```python
from build123d import *

# Parameters (mm, degrees)
F1_DEPTH = 1.27


with BuildPart() as f1:
    # F0 (on Front) → F1 (new body, symmetric)
    with BuildSketch(Plane.XZ):
        with BuildLine():
            Line((0, -4.572), (0, 0))
            Line((0, 0), (69.596, 0))
            Line((69.596, 0), (69.596, -4.572))
            Line((69.596, -4.572), (70.231, -4.572))
            Line((70.231, -4.572), (70.231, 0))
            ThreePointArc((70.231, 0), (70.0450128061, 0.4490128061), (69.596, 0.635))
            Line((69.596, 0.635), (0, 0.635))
            ThreePointArc((0, 0.635), (-0.4490128061, 0.4490128061), (-0.635, 0))
            Line((-0.635, 0), (-0.635, -4.572))
            Line((-0.635, -4.572), (0, -4.572))
        make_face()
    extrude(amount=F1_DEPTH, both=True)


solid = f1.part
```
The listing builds one solid part. Answer for the finished solid, in the listing's coordinates (mm). A direction names the side the tool comes from. Round coordinates to 2 decimals unless told otherwise and drop trailing zeros. Write each loop counter-clockwise with the first axis right and the second up, starting at its lowest first coordinate (ties: lowest second). Pieces come first, ordered by that corner, then holes. Notation, with made-up numbers: (61, 9.25) -> (120, 9.25) arc R26 ccw to (120, 48.25) -> close; hole circle Ø11 at (-15.5, 64.25). An arc over 180 degrees is marked (long way). Use CSV: the item, a comma, the result in double quotes. Start each with the question number.
(1) This flat-tipped pin is pushed along its axis until it touches: pin 1 (1.3 mm diameter, centred on x = 33.5, y = 0, fed in from -Z). Where does it stop, or does it pass through?
(2) Consider L1, parallel to X at y = -0.15, z = -3.4 (3 decimals); L2, parallel to Z at x = 30, y = 0.6 (3 decimals); L3, parallel to X at y = 1.1, z = 0.2. Determine where each line is inside the solid, lowest interval first. Write a range as from..to.
(3) Which of the six approach directions +Z, -Z, +X, -X, +Y, -Y give full straight-line access (tool end or side, diameter ignored) to faces 4 (the face through (0, 0, -2)), 5 (the face through (34.6, 1.27, 0.4))?
(4) Section B-B on y = -0.85 is taken. Give the vertices of the cut face in (x, z) (3 decimals).
(5) Section C-C on x = 16.5 is taken. Give the vertices of the cut face in (y, z) (3 decimals).
(6) Section A-A on z = -3.4 is taken. Give the vertices of the cut face in (x, y) (3 decimals).
(7) The mould has two halves that part along X. Classify faces 1 (the face through (70.231, 0, -2)), 2 (the face through (-0.635, 0, -2)), 3 (the face through (34, 0, 0)): released by +X, released by -X, zero draft, split by the parting line, or undercut.
A:
1,pin 1,"stops at z = 0"
2,L1,"x = -0.635..0, 69.596..70.231"
2,L2,"z = 0..0.635"
2,L3,"x = -0.6..70.2"
3,face 4,"-Z, +Y, -Y"
3,face 5,"+Z, -Z, +X, -X, +Y"
4,outline,"(-0.635, -4.572) -> (0, -4.572) -> (0, 0) -> (69.596, 0) -> (69.596, -4.572) -> (70.231, -4.572) -> (70.231, 0) arc R0.635 ccw to (69.596, 0.635) -> (0, 0.635) arc R0.635 ccw to (-0.635, 0) -> close"
5,outline,"(-1.27, 0) -> (1.27, 0) -> (1.27, 0.635) -> (-1.27, 0.635) -> close"
6,outline,"(-0.635, -1.27) -> (0, -1.27) -> (0, 1.27) -> (-0.635, 1.27) -> close; (69.596, -1.27) -> (70.231, -1.27) -> (70.231, 1.27) -> (69.596, 1.27) -> close"
7,face 1,"released by +X"
7,face 2,"released by -X"
7,face 3,"undercut"
